Here's how the part is built. I have some questions about the finished solid (model axes, mm). Face numbers are marked on the shaded views. Give positions to 0.01 mm unless a question says otherwise; leave off trailing zeros. Write each loop counter-clockwise with the first axis right and the second up, starting at its lowest first coordinate (ties: lowest second). Pieces come first, ordered by that corner, then holes. Notation, with made-up numbers: M 75,60.5 L 121,60.5 A19 ccw 121,97.5 Z; hole C 71.25,79 d3. An arc over 180 degrees is marked long. Use one line per item in the form item = value. Start each with the question number.
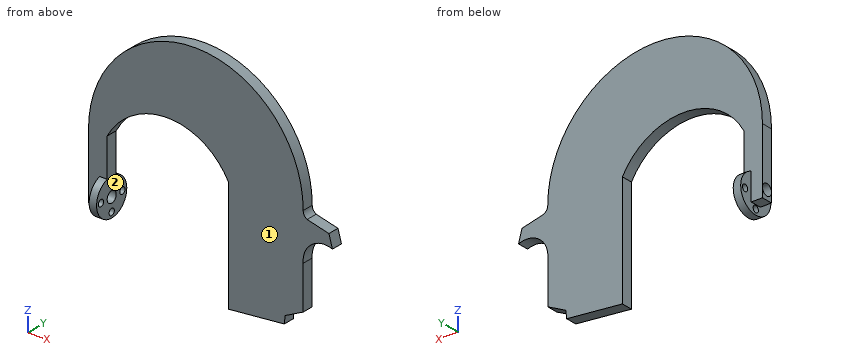
Autodesk Inventor part; units mm, degrees
ref_plane "YZ Plane" through (0, 0, 0) normal (1, 0, 0) x (0, 1, 0)
ref_plane "XZ Plane" through (0, 0, 0) normal (0, 1, 0) x (-1, 0, 0)
ref_plane "XY Plane" through (0, 0, 0) normal (0, 0, 1) x (1, 0, 0)
sketch "prindere" plane through (0, 0, 0) normal (0, 0, 1) x (1, 0, 0)
  circle A0 centre (0, 0) radius 10 construction
  circle A1 centre (0, -7.1) radius 1.75 construction
  circle A2 centre (0, 7.1) radius 1.75 construction
  circle A3 centre (-7.1, 0) radius 1.75 construction
  circle A4 centre (7.1, 0) radius 1.75 construction
  circle A5 centre (0, 0) radius 1.65 construction
  dimension "d1" = 10
sketch "Sketch1" plane through (0, 0, 0) normal (0, 1, 0) x (-1, 0, 0)
  line L0 (67.0192, 27.1113) -> (57.0192, 27.1113) construction
  line L1 (57.0192, 27.1113) -> (57.0192, -7.8887)
  line L2 (57.0192, -7.8887) -> (67.0192, -7.8887)
  line L3 (67.0192, -7.8887) -> (67.0192, 27.1113)
  line L4 (-7.9808, 27.1113) -> (-47.9808, 27.1113) construction
  line L5 (-47.9808, 27.1113) -> (-47.9808, -20.8435)
  line L6 (-47.9808, -32.8887) -> (-7.9808, -32.8887) construction
  line L7 (-7.9808, -32.8887) -> (-7.9808, 27.1113)
  arc A0 (57.0192, 27.1113) -> (-7.9808, 27.1113) centre (24.5192, 9.6227) ccw
  arc A1 (67.0192, 27.1113) -> (-47.9808, 27.1113) centre (9.5192, 27.1113) ccw
  arc A2 (-50.0815, 23.591) -> (-47.9808, 27.1113) centre (-51.9808, 27.1113) ccw
  line L8 (-50.0815, 23.591) -> (-61.765, 20.853)
  line L9 (-61.765, 20.853) -> (-63.6478, 14.111)
  arc A3 (-47.9808, 2.187) -> (-63.6478, 14.111) centre (-59.4808, 3.3315) ccw
  line L10 (-7.9808, -32.8887) -> (-37.8292, -29.876)
  line L11 (-37.8292, -29.876) -> (-38.3378, -25.7069)
  line L12 (-38.3378, -25.7069) -> (-47.9808, -20.8435)
  line L13 (-47.9808, -20.8435) -> (-47.9808, -32.8887) construction
  point P0 (0, 0)
  dimension "d0" = 35
  dimension "d1" = 10
  dimension "d2" = 60
  dimension "d3" = 40
  dimension "d4" = 65
  dimension "d5" = 36.9066
  dimension "d6" = 12
  dimension "d7" = 4
  dimension "d8" = 7
  dimension "d9" = 11.5
  dimension "d10" = 30
  dimension "d11" = 10.8
  dimension "d12" = 4.2
  dimension "d13" = 11.5568
  dimension "d14" = 84.237
  dimension "d15" = 6.957
  dimension "d16" = 76.811
  dimension "d17" = 15.603
  dimension "d18" = 67.0192
  dimension "d19" = 7.8887
  dimension "d20" = 34.3956
extrude "Extrusion1" add sketch "Sketch1" along normal blind 6 contours A0 L7 L10 L11 L12 L5 A3 A1 L3 L2 L1 | L5 A3 L9 L8 A2
sketch "Sketch2" plane through (-57.0192, 0, 27.1113) normal (1, 0, 0) x (0, 0, -1)
  line L0 (0, 0) -> (35, 0) construction
  line L1 (35, 0) -> (35, 6) construction
  line L2 (0, 6) -> (35, 6) construction
  line L3 (0, 0) -> (0, 6) construction
  line L4 (0, 0) -> (0, 6) construction
  line L5 (0, 3) -> (35, 3) construction
  circle A0 centre (30, 3) radius 10
  circle A1 centre (30, 10.1) radius 1.75
  circle A2 centre (37.1, 3) radius 1.75
  circle A3 centre (30, -4.1) radius 1.75
  circle A4 centre (30, 3) radius 1.65
  point P0 (27.1113, 0)
  dimension "d23" = 5
extrude "Extrusion2" add sketch "Sketch2" against normal blind 4
sketch "Sketch3" plane through (-57.0192, 0, 27.1113) normal (1, 0, 0) x (0, 0, -1)
  arc A0 (20.4606, 0) -> (20.4606, 6) centre (30, 3) ccw
  circle A1 centre (30, 3) radius 3
  point P0 (27.1113, 0)
  dimension "d26" = 6
extrude "Extrusion3" cut sketch "Sketch3" against normal through all
equation "\"d1\" = hmic"
equation "\"d0\" = lmic"
equation "\"d2\" = lmare"
equation "\"d3\" = hmare"
equation "\"d4\" = rcerc"
equation "\"d6\" = laripa"
equation "\"d7\" = rcerculet1"
equation "\"d8\" = haripa"
equation "\"d9\" = rcerculet2"
equation "\"d10\" = 0.5 * lmare"
equation "\"d11\" = 0.18 * lmare"
equation "\"d12\" = 0.07 * lmare"
equation "\"d21\" = grosime"
equation "\"lmic\" = 35"
equation "\"hmic\" = 10"
equation "\"rcerc\" = 65"
equation "\"lmare\" = 60"
equation "\"hmare\" = 40"
equation "\"rcerculet1\" = 4"
equation "\"rcerculet2\" = 11.5"
equation "\"laripa\" = 12"
equation "\"haripa\" = 7"
equation "\"grosime\" = 6"
properties part number "carma"
1) Suppose I cut it at A-A, the plane z = 44. List the corners of the cut face in (x, y) for me, and give its area (3 significant figures).
2) Thinking about a two-plate mould opening in X: for the marked faces 1 and 2, which applies, released by +X, released by -X, zero draft, split by the parting line, or undercut?
3) Suppose I cut it at D-D, the plane z = 66. List the corners of the cut face in (x, y) for me.
4) Please list where these lines run through material, in increasing order: line 1 (X direction, y = 2.25, z = 27); line 2 (Y direction, x = 23, z = 7.5); line 3 (X direction, y = 0.5, z = 37).
5) Will these pins go through, and if not, where does the flat tip stop? P1, Ø1, axis at x = 6, y = 6, coming from the -Z side; P2, Ø12, axis at x = 30, z = -20.5, coming from the -Y side; P3, Ø10, axis at y = 1.5, z = 69, coming from the +X side.
6) Suppose I cut it at B-B, the plane y = 3. State how many separate pieces and enclosed holes the cut face has, and give its area (3 significant figures).
7) Suppose I cut it at C-C, the plane y = 10.1. List the corners of the cut face in (x, z) for me.
Checks:
q1.outline = M -64.48,0 L -37.95,0 L -37.95,6 L -64.48,6 Z; M -11.09,0 L 45.44,0 L 45.44,6 L -11.09,6 Z
q1.area = 498 mm^2
q2.face_1 = zero draft
q2.face_2 = undercut
q3.outline = M -51.87,0 L 32.84,0 L 32.84,6 L -51.87,6 Z
q4.line_1 = -67.02 to -57.02, 7.98 to 47.98
q4.line_2 = 0 to 6
q4.line_3 = -66.16 to -49.27, 0.23 to 47.12
q5.P1 = 29.62
q5.P2 = 0
q5.P3 = 34.59
q6.separate_pieces = 3
q6.enclosed_holes = 0
q6.area = 6,990 mm^2
q7.outline = M -61.02,-9.93 L -57.02,-9.93 L -57.02,-4.64 L -61.02,-4.64 Z; M -61.02,-1.14 L -57.02,-1.14 L -57.02,4.15 L -61.02,4.15 Z
